from build123d import *
from build123d.topology import SkipClean

# Parameters (mm, degrees)
BOSS_EXTRU_1_DEPTH       = 20
ESQUISSE4_R              = 22.5
BOSS_EXTRU_2_DEPTH       = 26.35
ESQUISSE6_R              = 9.5
ENL_V_MAT_EXTRU_1_DEPTH  = 174.395073781
ENL_V_MAT_EXTRU_2_DEPTH  = 9.5
CONG_1_R                 = 7.5
ENL_V_START              = -9.5
ENL_V_MAT_EXTRU_10_DEPTH = 9.5
ENL_V_MAT_EXTRU_6_DEPTH  = 9.5
CONG_3_R                 = 7.5
ENL_V_MAT_EXTRU_7_DEPTH  = 9.5
CONG_4_R                 = 7.5
BOSS_EXTRU_4_DEPTH       = 18.5
ESQUISSE14_R             = 8
ENL_V_MAT_EXTRU_8_DEPTH  = 146.629175394
BOSS_EXTRU_5_DEPTH       = 18.5
ESQUISSE16_R             = 8
ENL_V_MAT_EXTRU_9_DEPTH  = 171.14276454


with BuildPart() as part:
    # Esquisse2 → Boss.-Extru.1 (new, symmetric)
    with BuildSketch(Plane.XY):
        with BuildLine():
            Line((0, 0), (88.25, 0))
            ThreePointArc((88.25, 0), (69.01448291, 34.172398309), (108.207743747, 32.889343798))
            Line((108.207743747, 32.889343798), (71.268065021, 103.849806406))
            Line((71.268065021, 103.849806406), (59.515171481, 97.731637281))
            Line((59.515171481, 97.731637281), (46.585999978, 122.568344656))
            Line((46.585999978, 122.568344656), (30.176299564, 114.025995311))
            Line((30.176299564, 114.025995311), (43.105471067, 89.189287936))
            Line((43.105471067, 89.189287936), (0, 66.75))
            Line((0, 66.75), (0, 31.75))
            Line((0, 31.75), (-31.75, 31.75))
            Line((-31.75, 31.75), (-31.75, 13.25))
            Line((-31.75, 13.25), (0, 13.25))
            Line((0, 13.25), (0, 0))
        make_face()
    extrude(amount=BOSS_EXTRU_1_DEPTH, both=True)

    # Esquisse4 → Boss.-Extru.2 (add, symmetric)
    with BuildSketch(Plane.XY):
        with Locations((88.25, 22.5)):
            Circle(ESQUISSE4_R)
    extrude(amount=BOSS_EXTRU_2_DEPTH, both=True)

    # Esquisse6 → Enlèv. mat.-Extru.1 (cut, through all)
    with BuildSketch(Plane.XY.offset(26.35)):
        with Locations((88.25, 22.5)):
            Circle(ESQUISSE6_R)
    extrude(amount=-ENL_V_MAT_EXTRU_1_DEPTH, mode=Mode.SUBTRACT)

    # Esquisse7 → Enlèv. mat.-Extru.2 (cut)
    with SkipClean():  # the faces are left unmerged after this step: merging them gives an invalid solid
        with BuildSketch(Plane.XY.offset(20)):
            with BuildLine():
                Line((9.5, 0), (9.5, 13.25))
                Line((9.5, 13.25), (63.361498639, 13.25))
                ThreePointArc((63.361498639, 13.25), (66.885966684, 12.370281338), (69.583623979, 9.9375))
                ThreePointArc((69.583623979, 9.9375), (77.676595865, 2.639155985), (88.25, 0))
                Line((88.25, 0), (9.5, 0))
            make_face()
        extrude(amount=-ENL_V_MAT_EXTRU_2_DEPTH, mode=Mode.SUBTRACT)

    # Congé1
    cong_1_edges = [part.edges().sort_by_distance(p)[0] for p in [
        (9.5, 13.25, 15.25),
    ]]
    fillet(cong_1_edges, radius=CONG_1_R)

    # Esquisse18 → Enlèv. mat.-Extru.10 (cut)
    with BuildSketch(Plane(origin=(0, 0, -20), x_dir=(-1, 0, 0), z_dir=(0, 0, -1)).offset(ENL_V_START)):
        with BuildLine():
            Line((-9.5, 0), (-88.25, 0))
            ThreePointArc((-88.25, 0), (-77.676595865, 2.639155985), (-69.583623979, 9.9375))
            ThreePointArc((-69.583623979, 9.9375), (-66.885966684, 12.370281338), (-63.361498639, 13.25))
            Line((-63.361498639, 13.25), (-9.5, 13.25))
            Line((-9.5, 13.25), (-9.5, 0))
        make_face()
    extrude(amount=ENL_V_MAT_EXTRU_10_DEPTH, mode=Mode.SUBTRACT)

    # Esquisse11 → Enlèv. mat.-Extru.6 (cut)
    with BuildSketch(Plane.XY.offset(20)):
        with BuildLine():
            Line((47.492082893, 80.762685021), (67.299435542, 42.713114599))
            ThreePointArc((67.299435542, 42.713114599), (67.058693323, 35.359200564), (60.646854293, 31.75))
            Line((60.646854293, 31.75), (9.5, 31.75))
            Line((9.5, 31.75), (9.5, 60.985258485))
            Line((9.5, 60.985258485), (47.492082893, 80.762685021))
        make_face()
        with BuildLine():
            Line((63.901783307, 89.305034366), (84.962619218, 48.847545001))
            ThreePointArc((84.962619218, 48.847545001), (87.370357433, 46.127512536), (90.77390035, 44.8579947))
            ThreePointArc((90.77390035, 44.8579947), (100.984529101, 41.049441193), (108.207743747, 32.889343798))
            Line((108.207743747, 32.889343798), (75.654676846, 95.423203491))
            Line((75.654676846, 95.423203491), (63.901783307, 89.305034366))
        make_face()
    extrude(amount=-ENL_V_MAT_EXTRU_6_DEPTH, mode=Mode.SUBTRACT)

    # Congé3
    cong_3_edges = [part.edges().sort_by_distance(p)[0] for p in [
        (63.901783307, 89.305034366, 15.25),
        (9.5, 60.985258485, 15.25),
        (47.492082893, 80.762685021, 15.25),
        (9.5, 31.75, 15.25),
    ]]
    fillet(cong_3_edges, radius=CONG_3_R)

    # Esquisse12 → Enlèv. mat.-Extru.7 (cut)
    with BuildSketch(Plane(origin=(0, 0, -20), x_dir=(-1, 0, 0), z_dir=(0, 0, -1)).offset(ENL_V_START)):
        with BuildLine():
            Line((-75.654676846, 95.423203491), (-108.207743747, 32.889343798))
            ThreePointArc((-108.207743747, 32.889343798), (-100.984529101, 41.049441193), (-90.77390035, 44.8579947))
            ThreePointArc((-90.77390035, 44.8579947), (-87.370357433, 46.127512536), (-84.962619218, 48.847545001))
            Line((-84.962619218, 48.847545001), (-63.901783307, 89.305034366))
            Line((-63.901783307, 89.305034366), (-75.654676846, 95.423203491))
        make_face()
        with BuildLine():
            Line((-9.5, 31.75), (-9.5, 60.985258485))
            Line((-9.5, 60.985258485), (-47.492082893, 80.762685021))
            Line((-47.492082893, 80.762685021), (-67.299435542, 42.713114599))
            ThreePointArc((-67.299435542, 42.713114599), (-67.058693323, 35.359200564), (-60.646854293, 31.75))
            Line((-60.646854293, 31.75), (-9.5, 31.75))
        make_face()
    extrude(amount=ENL_V_MAT_EXTRU_7_DEPTH, mode=Mode.SUBTRACT)

    # Congé4
    cong_4_edges = [part.edges().sort_by_distance(p)[0] for p in [
        (9.5, 31.75, -15.25),
        (47.492082893, 80.762685021, -15.25),
        (9.5, 60.985258485, -15.25),
        (63.901783307, 89.305034366, -15.25),
    ]]
    fillet(cong_4_edges, radius=CONG_4_R)

    # Esquisse13 → Boss.-Extru.4 (add)
    with BuildSketch(Plane(origin=(0, 31.75, 0), x_dir=(1, 0, 0), z_dir=(0, 1, 0))):
        with BuildLine():
            Line((-31.75, -20), (-31.75, 20))
            ThreePointArc((-31.75, 20), (-51.75, 0), (-31.75, -20))
        make_face()
    extrude(amount=-BOSS_EXTRU_4_DEPTH)

    # Esquisse14 → Enlèv. mat.-Extru.8 (cut, through all)
    with BuildSketch(Plane(origin=(0, 31.75, 0), x_dir=(1, 0, 0), z_dir=(0, 1, 0))):
        with Locations(Location((-31.75, 0, 0), (0, 0, 270))):
            Circle(ESQUISSE14_R)
    extrude(amount=-ENL_V_MAT_EXTRU_8_DEPTH, mode=Mode.SUBTRACT)

    # Esquisse15 → Boss.-Extru.5 (add)
    with BuildSketch(Plane(origin=(86.854370959, 45.213523718, 0), x_dir=(0, 0, -1), z_dir=(0.8870108331782227, 0.4617486132350318, 0))):
        with BuildLine():
            Line((-20, 87.208428629), (20, 87.208428629))
            ThreePointArc((20, 87.208428629), (0, 107.208428629), (-20, 87.208428629))
        make_face()
    extrude(amount=-BOSS_EXTRU_5_DEPTH)

    # Esquisse16 → Enlèv. mat.-Extru.9 (cut, through all)
    with BuildSketch(Plane(origin=(86.854370959, 45.213523718, 0), x_dir=(0, 0, -1), z_dir=(0.8870108331782227, 0.4617486132350318, 0))):
        with Locations(Location((0, 87.208428629, 0), (0, 0, 90))):
            Circle(ESQUISSE16_R)
    extrude(amount=-ENL_V_MAT_EXTRU_9_DEPTH, mode=Mode.SUBTRACT)


solid = part.part
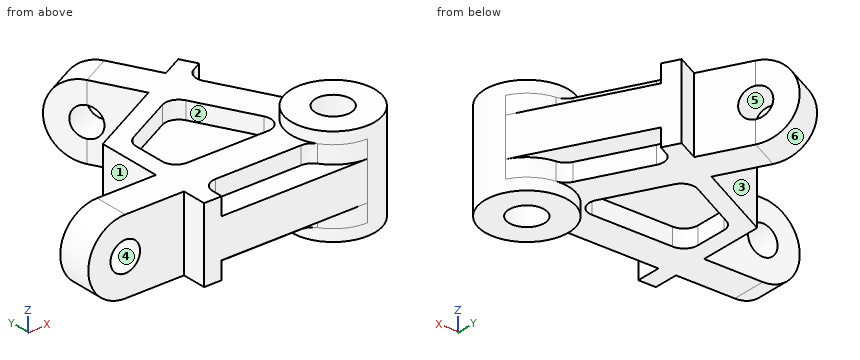
Model file for the job. Use its own axes, mm. Face numbers are marked on the shaded views. A direction names the side the tool comes from. Round coordinates to 2 decimals unless told otherwise and drop trailing zeros. Loops run counter-clockwise (first coordinate to the right, second up) from the corner with the lowest first, then second, coordinate; pieces in that order, holes last. Notation, with made-up numbers: (-9, 7) - (29, 7) arc R22 ccw to (29, 36) - close; hole circle Ø10 at (21.25, 63). An arc over 180 degrees is marked (long way). Write each question's results on one line, items separated by ' | '.
(1) Saw through at C-C, the plane z = -13. Count the separate pieces of the cut face and the enclosed holes in it, then the cut area to 3 significant figures.
Answer below:
separate pieces: 1 | enclosed holes: 2 | area: 6,340 mm^2
(2) Saw through at B-B, the plane z = -4. List the corners of the cut face in (x, y).
Answer below:
outline: (-51.35, 13.25) - (-38.68, 13.25) - (-38.68, 31.75) - (-51.35, 31.75) - close; (-24.82, 13.25) - (0, 13.25) - (0, 0) - (88.25, 0) arc R22.5 ccw to (108.21, 32.89) - (71.27, 103.85) - (59.52, 97.73) - (49.79, 116.42) - (33.38, 107.88) - (43.11, 89.19) - (0, 66.75) - (0, 31.75) - (-24.82, 31.75) - close; (21.13, 131.41) - (26.98, 120.17) - (43.39, 128.71) - (37.54, 139.95) - close; hole circle Ø19 at (88.25, 22.5)
(3) 3-axis set-ups, long thin cutter, end or side, ignore diameter. For the marked faces 1, 2 and 3: which of +Z, -Z, +X, -X, +Y, -Y reach the whole face in a straight line?
Answer below:
face 1: +Z, -Z, -X, +Y | face 2: +Z | face 3: +Z, -Z, -X
(4) Wall check: L1, parallel to X at y = 23.25, z = 0; L2, parallel to Y at x = 41.5, z = -11.5; L3, parallel to Y at x = 88.25, z = -0.5. Give the ranges that are in metal, low to high.
Answer below:
L1: x = -51.75 to -39.75, -23.75 to 78.78, 97.72 to 110.74 | L2: y = 13.25 to 31.75, 77.6 to 88.35, 92.27 to 132.34 | L3: y = 0 to 13, 32 to 71.23
(5) Mould opens along Y. For the marked faces 4, 5 and 6 say: released by +Y, released by -Y, zero draft, split by the parting line, or undercut.
Answer below:
face 4: zero draft | face 5: undercut | face 6: released by +Y
(6) Saw through at A-A, the plane y = 22.5. List the corners of the cut face in (x, z).
Answer below:
outline: (-31.75, -20) - (65.75, -20) - (65.75, -26.35) - (78.75, -26.35) - (78.75, 26.35) - (65.75, 26.35) - (65.75, 20) - (-31.75, 20) arc R20 ccw to start; (97.75, -26.35) - (110.75, -26.35) - (110.75, 26.35) - (97.75, 26.35) - close; hole circle Ø16 at (-31.75, 0)
(7) Saw through at D-D, the plane z = 5.5. List the corners of the cut face in (x, y), then the cut area to 3 significant figures.
Answer below:
outline: (-50.98, 13.25) - (-37.56, 13.25) - (-37.56, 31.75) - (-50.98, 31.75) - close; (-25.94, 13.25) - (0, 13.25) - (0, 0) - (88.25, 0) arc R22.5 ccw to (108.21, 32.89) - (71.27, 103.85) - (59.52, 97.73) - (49.27, 117.42) - (32.86, 108.87) - (43.11, 89.19) - (0, 66.75) - (0, 31.75) - (-25.94, 31.75) - close; (21.3, 131.08) - (27.49, 119.18) - (43.9, 127.72) - (37.71, 139.62) - close; hole circle Ø19 at (88.25, 22.5) | area: 9,670 mm^2
(8) Pin check, flat tips, straight feed: pin 1 (6 mm diameter, centred on x = 22, y = 47.5, fed in from -Z); pin 2 (20 mm diameter, centred on x = -23, z = -2.5, fed in from +Y); pin 3 (3 mm diameter, centred on y = 25.5, z = 5.5, fed in from -X). Stop position of each tip, or through.
Answer below:
pin 1: stops at z = -10.5 | pin 2: stops at y = 31.75 | pin 3: stops at x = -51.35
